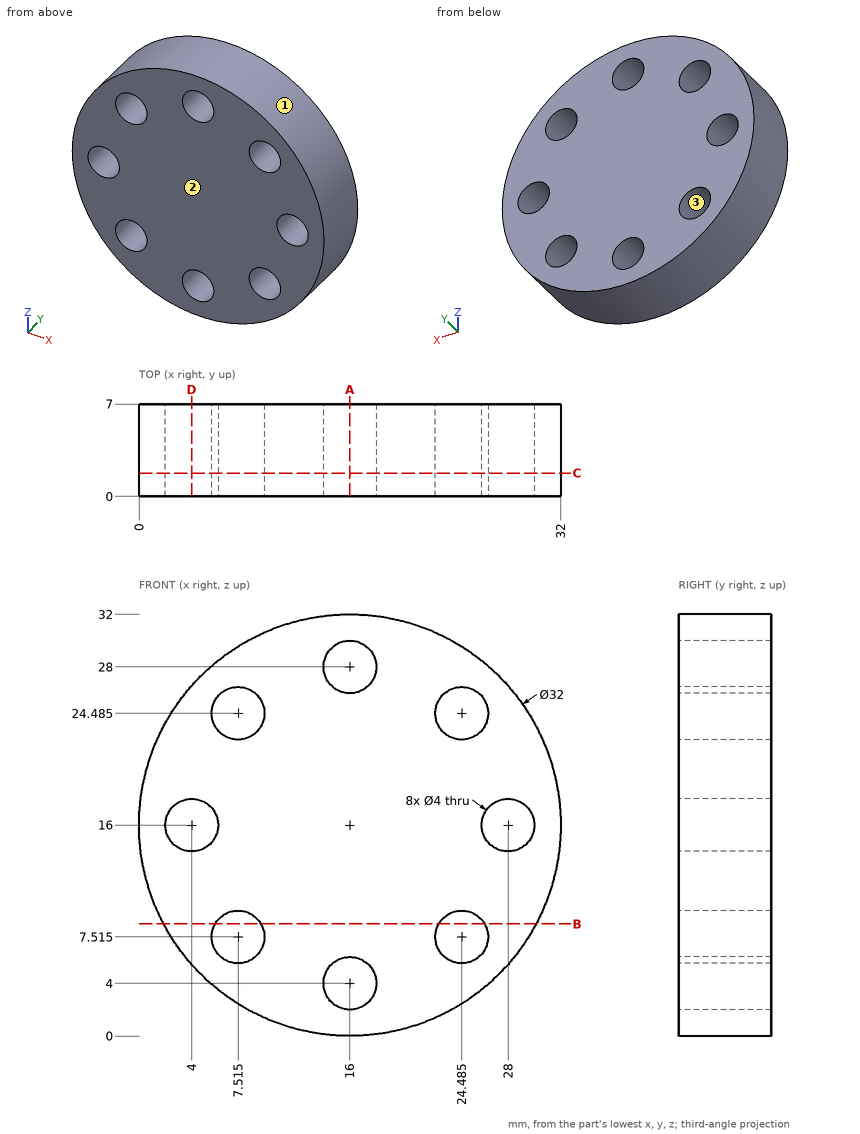
Check sheet for the drawn part. Datum: minimum x, y, z corner. Units: mm. Round coordinates to 2 decimals unless told otherwise and drop trailing zeros. Write each loop counter-clockwise with the first axis right and the second up, starting at its lowest first coordinate (ties: lowest second). Pieces come first, ordered by that corner, then holes. Notation, with made-up numbers: (48.5, -35) -> (95.5, -35) arc R19 cw to (95.5, -7) -> close; hole circle Ø5 at (75.25, -7). An arc over 180 degrees is marked (long way). One line per item, written item: value. Start each with the question number.
(1) Cross-section at B-B, the plane z = 8.5. Record the cut outline in (x, y) (1 decimal).
(2) Go/stop test with flat-tipped pins: pin 1 Ø4 at (x, y) = (26.5, 2.5) entering from +Z (1 decimal); pin 2 Ø3 at (y, z) = (2, 22.5) entering from -X; pin 3 Ø3 at (x, y) = (19, 1) entering from -Z. Record where each tip stops, or that it passes through.
(3) Cross-section at D-D, the plane x = 4. Record the cut outline in (y, z), and give its area (3 significant figures).
(4) Scan lines: line 1 (Z direction, x = 14.5, y = 3.5); line 2 (X direction, y = 6, z = 7). Record each from-to range of solid material in increasing order. Write a range as [from, to].
(5) Cross-section at C-C, the plane y = 1.75. Give the number of separate pieces and of enclosed holes in the cut face, and give its area (3 significant figures).
(6) Cross-section at A-A, the plane x = 16. Record the cut outline in (y, z), and give its area (3 significant figures).
(7) Draft check along X on the marked faces 1, 2 and 3. Enter one of: +X half, -X half, draft (parallel to the pull), parting line (faces both ways), or undercut.
Answer:
1. outline: (1.9, 0) -> (5.8, 0) -> (5.8, 7) -> (1.9, 7) -> close; (9.3, 0) -> (22.7, 0) -> (22.7, 7) -> (9.3, 7) -> close; (26.2, 0) -> (30.1, 0) -> (30.1, 7) -> (26.2, 7) -> close
2. pin 1: z = 29.6
2. pin 2: x = 0.8
2. pin 3: z = 0.07
3. outline: (0, 5.42) -> (7, 5.42) -> (7, 14) -> (0, 14) -> close; (0, 18) -> (7, 18) -> (7, 26.58) -> (0, 26.58) -> close
3. area: 120 mm²
4. line 1: [0.07, 2.68], [5.32, 26.68], [29.32, 31.93]
4. line 2: [2.77, 5.58], [9.45, 22.55], [26.42, 29.23]
5. separate pieces: 1
5. enclosed holes: 8
5. area: 704 mm²
6. outline: (0, 0) -> (7, 0) -> (7, 2) -> (0, 2) -> close; (0, 6) -> (7, 6) -> (7, 26) -> (0, 26) -> close; (0, 30) -> (7, 30) -> (7, 32) -> (0, 32) -> close
6. area: 168 mm²
7. face 1: parting line
7. face 2: draft
7. face 3: undercut
